```python
from build123d import *

# Parameters (mm, degrees)
PAD_DEPTH    = 40
SKETCH_R     = 5
POCKET_DEPTH = 50.001


with BuildPart() as part:
    # Sketch001 → Pad (new body)
    with BuildSketch(Plane.XZ):
        with BuildLine():
            Line((0, 0), (110, 0))
            Line((110, 0), (110, 27.159005))
            ThreePointArc((110, 27.159005), (105.316047, 43.099238), (90.20281, 50))
            Line((50, 50), (90.20281, 50))
            Line((0, 21.132487), (50, 50))
            Line((0, 0), (0, 21.132487))
        make_face()
    extrude(amount=-PAD_DEPTH)

    # Sketch (on Face4 of Pad) → Pocket (cut, through all)
    with BuildSketch(Plane(origin=(0, 0, 50), x_dir=(-1, 0, 0), z_dir=(0, 0, 1))):
        with Locations((-69.999992, -20.000006)):
            Circle(SKETCH_R)
    extrude(amount=-POCKET_DEPTH, mode=Mode.SUBTRACT)


solid = part.part
```
Geometry check sheet. Reference: the model listing, model coordinates, mm. A direction names the side the tool comes from. Round coordinates to 2 decimals unless told otherwise and drop trailing zeros. Loops run counter-clockwise (first coordinate to the right, second up) from the corner with the lowest first, then second, coordinate; pieces in that order, holes last. Notation, with made-up numbers: (38.5, -17) - (60.5, -17) arc R31 cw to (60.5, 18) - close; hole circle Ø11 at (-11, -1). An arc over 180 degrees is marked (long way). Write each question's results on one line, items separated by ' | '. Start each with the question number.
Q1. Gauge pin test, flat ends, axial feed: P1, Ø6, axis at x = 25, y = 35.5, coming from the +Z side; P2, Ø5, axis at x = 22.5, y = 9, coming from the +Z side; P3, Ø2, axis at y = 22.5, z = 24, coming from the -X side; P4, Ø8, axis at x = 28.5, z = 23, coming from the -Y side. Record the tip position at first contact, or that the pin passes through.
Q2. Cross-section at A-A on x = 68. Enter the section's corners in (y, z).
Q3. Cross-section at C-C on y = 27. Enter the section's corners in (x, z).
Q4. Cross-section at D-D on z = 30. Enter the section's corners in (x, y), and give its area (3 significant figures).
Q5. Cross-section at B-B on z = 14. Enter the section's corners in (x, y), and give its area (3 significant figures).
Q6. Access from +Z, -Z, +X, -X, +Y, -Y to the whole of each face (thin tool, end or side, straight path). Record for faces 5 (the flat face through (0, 20, 10)), 6 (the flat face through (110, 20, 13)).
Q7. Thickness scan on line 1 (X direction, y = 7, z = 5); line 2 (X direction, y = 21, z = 5.5); line 3 (X direction, y = 22.5, z = 30). Record the ranges inside material, lowest first. Write a range as [from, to].
Q8. Release check for a two-part mould opening along Y. For faces 1 (the flat face through (54, 40, 25)), 2 (the flat face through (24.65, 19.72, 35.364)), 3 (the flat face through (54, 0, 25)), 4 (the cylindrical face through (65.381, 21.915, 25.35)) record: +Y half, -Y half, draft (parallel to the pull), parting line (faces both ways), or undercut.
Answers below:
1) P1: stops at z = 37.3 | P2: stops at z = 35.57 | P3: stops at x = 3.23 | P4: stops at y = 0
2) outline: (0, 0) - (15.42, 0) - (15.42, 50) - (0, 50) - close; (24.58, 0) - (40, 0) - (40, 50) - (24.58, 50) - close
3) outline: (0, 0) - (110, 0) - (110, 27.16) arc R20 ccw to (90.2, 50) - (50, 50) - (0, 21.13) - close
4) outline: (15.36, 0) - (110.2, 0) - (110.2, 40) - (15.36, 40) - close; hole circle Ø10 at (70, 20) | area: 3,720 mm²
5) outline: (0, 0) - (110, 0) - (110, 40) - (0, 40) - close; hole circle Ø10 at (70, 20) | area: 4,320 mm²
6) face 5: +Z, -Z, -X, +Y, -Y | face 6: -Z, +X, +Y, -Y
7) line 1: x = [0, 110] | line 2: x = [0, 65.1], [74.9, 110] | line 3: x = [15.36, 65.67], [74.33, 110.2]
8) face 1: +Y half | face 2: draft | face 3: -Y half | face 4: undercut
